Part model, mm, in its own coordinate system. Face numbers are marked on the shaded views. A direction names the side the tool comes from. Round coordinates to 2 decimals unless told otherwise and drop trailing zeros. Loops run counter-clockwise (first coordinate to the right, second up) from the corner with the lowest first, then second, coordinate; pieces in that order, holes last.
1) Drop flat-ended pins along their axis: P1, Ø3, axis at x = -4.5, y = 4.5, coming from the +Z side; P2, Ø10, axis at x = -6, z = 37, coming from the -Y side. Give the stop position or say it passes through.
2) Band-saw the part on C-C, the plane y = 5.75. Write the cut outline in (x, z), then the cut area to 3 significant figures.
3) Probe line 1 (Z direction, x = 0.25, y = 6.25); line 2 (Y direction, x = -2.5, z = 27.5). List the from-to ranges inside material, lowest first.
4) Band-saw the part on B-B, the plane z = 31. Write the cut outline in (x, y).
5) Band-saw the part on A-A, the plane x = 4. Write the cut outline in (y, z), then the cut area to 3 significant figures.
6) 3-axis set-ups, long thin cutter, end or side, ignore diameter. For the marked faces 1 and 2: which of +Z, -Z, +X, -X, +Y, -Y reach the whole face in a straight line?
from build123d import *

# Parameters (mm, degrees)
F0_W     = 20
F0_H     = 20
F0_H_2   = 50
F1_DEPTH = 20
F2_DEPTH = 10


with BuildPart() as f1:
    # F0 (on Front) → F1 (new body)
    with BuildSketch(Plane.XZ):
        with Locations((-4.364679, 34.713301)):
            Rectangle(F0_W, F0_H)
        with Locations((-4.364679, -0.286699)):
            Rectangle(F0_W, F0_H_2)
    extrude(amount=-F1_DEPTH)

    # F0 (on Front) → F2 (cut)
    with BuildSketch(Plane.XZ):
        with Locations((-4.364679, 34.713301)):
            Rectangle(F0_W, F0_H)
    extrude(amount=-F2_DEPTH, mode=Mode.SUBTRACT)


solid = f1.part
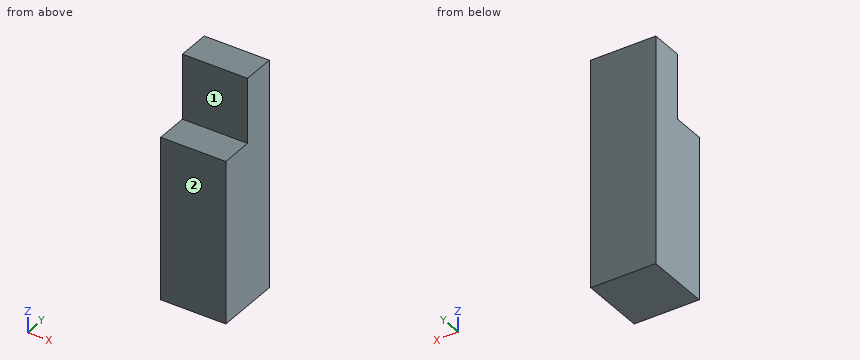
Reported:
1. P1: stops at z = 24.71
1. P2: stops at y = 10
2. outline: (-14.36, -25.29) - (5.64, -25.29) - (5.64, 24.71) - (-14.36, 24.71) - close
2. area: 1,000 mm2
3. line 1: z = -25.29 to 24.71
3. line 2: y = 10 to 20
4. outline: (-14.36, 10) - (5.64, 10) - (5.64, 20) - (-14.36, 20) - close
5. outline: (0, -25.29) - (20, -25.29) - (20, 44.71) - (10, 44.71) - (10, 24.71) - (0, 24.71) - close
5. area: 1,200 mm2
6. face 1: +Z, +X, -X, -Y
6. face 2: +Z, -Z, +X, -X, -Y
